Here's how the part is built. I have some questions about the finished solid (model axes, mm). Face numbers are marked on the shaded views. A direction names the side the tool comes from. Give positions to 0.01 mm unless a question says otherwise; leave off trailing zeros. Loops run counter-clockwise (first coordinate to the right, second up) from the corner with the lowest first, then second, coordinate; pieces in that order, holes last. Notation, with made-up numbers: (13, -38) - (51, -38) arc R25 cw to (51, -17) - close; hole circle Ø4 at (62.5, 85). An arc over 180 degrees is marked (long way). Use a Markdown table: item, result.
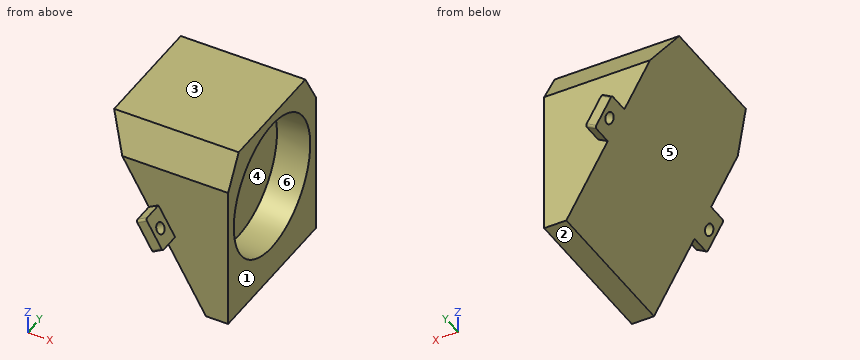
from build123d import *

# Parameters (mm, degrees)
BOSS_EXTRUDE1_DEPTH = 88.9
SKETCH2_R           = 38.735
CUT_EXTRUDE1_DEPTH  = 6.35
SKETCH3_W           = 101.6
SKETCH3_H           = 88.9
SKETCH3_R           = 38.735
BOSS_EXTRUDE2_DEPTH = 12.7
BOSS_EXTRUDE4_DEPTH = 12.7
SKETCH6_R           = 3.175
CUT_EXTRUDE2_DEPTH  = 58.15
BOSS_EXTRUDE5_DEPTH = 12.7
SKETCH8_R           = 3.175
CUT_EXTRUDE3_DEPTH  = 58.15
FILLET1_R           = 1.27
CUT_EXTRUDE4_DEPTH  = 72.35878735


with BuildPart() as part:
    # Sketch1 → Boss-Extrude1 (new body)
    with BuildSketch(Plane(origin=(0, 0, 0), x_dir=(1, 0, 0), z_dir=(0, 1, 0))):
        Polygon((0, 0), (0, 101.6), (-58.65878735, 0), align=None)
    extrude(amount=BOSS_EXTRUDE1_DEPTH)

    # Sketch2 → Cut-Extrude1 (cut)
    with BuildSketch(Plane(origin=(0, 0, 0), x_dir=(0, 0, -1), z_dir=(1, 0, 0))):
        with Locations((44.45, 44.45)):
            Circle(SKETCH2_R)
    extrude(amount=-CUT_EXTRUDE1_DEPTH, mode=Mode.SUBTRACT)

    # Sketch3 → Boss-Extrude2 (add)
    with BuildSketch(Plane(origin=(0, 0, 0), x_dir=(0, 0, -1), z_dir=(1, 0, 0))):
        with Locations((50.8, 44.45)):
            Rectangle(SKETCH3_W, SKETCH3_H)
        with Locations((44.45, 44.45)):
            Circle(SKETCH3_R, mode=Mode.SUBTRACT)
    extrude(amount=BOSS_EXTRUDE2_DEPTH)

    # Sketch5 → Boss-Extrude4 (add)
    with BuildSketch(Plane.XZ):
        Polygon((-23.197585425, -61.42060343), (-32.722585425, -44.922819488), (-27.223324111, -41.747819488), (-17.698324111, -58.24560343), align=None)
    extrude(amount=BOSS_EXTRUDE4_DEPTH)

    # Sketch6 → Cut-Extrude2 (cut, through all)
    with BuildSketch(Plane(origin=(-38.494829198, 0, -22.225), x_dir=(0.5, 0, -0.866025404), z_dir=(0.866025404, 0, 0.5))):
        with Locations((32.068010174, -6.46367916)):
            Circle(SKETCH6_R)
    extrude(amount=-CUT_EXTRUDE2_DEPTH, mode=Mode.SUBTRACT)

    # Sketch7 → Boss-Extrude5 (add)
    with BuildSketch(Plane(origin=(0, 88.9, 0), x_dir=(1, 0, 0), z_dir=(0, 1, 0))):
        Polygon((-23.73378735, 60.491874454), (-18.234526036, 57.316874454), (-27.759526036, 40.819090512), (-33.25878735, 43.994090512), align=None)
    extrude(amount=BOSS_EXTRUDE5_DEPTH)

    # Sketch8 → Cut-Extrude3 (cut, through all)
    with BuildSketch(Plane(origin=(-38.494829198, 0, -22.225), x_dir=(0.5, 0, -0.866025404), z_dir=(0.866025404, 0, 0.5))):
        with Locations((30.995606325, 95.541359592)):
            Circle(SKETCH8_R)
    extrude(amount=-CUT_EXTRUDE3_DEPTH, mode=Mode.SUBTRACT)

    # Fillet1
    fillet1_edges = [part.edges().sort_by_distance(p)[0] for p in [
        (-20.447954768, -12.7, -59.83310343),
        (-29.972954768, -12.7, -43.335319488),
        (-30.509156693, 101.6, -42.406590512),
        (-20.984156693, 101.6, -58.904374454),
    ]]
    fillet(fillet1_edges, radius=FILLET1_R)

    # Sketch9 → Cut-Extrude4 (cut, through all)
    with BuildSketch(Plane(origin=(12.7, 0, 0), x_dir=(0, 0, -1), z_dir=(1, 0, 0))):
        Polygon((18.509160794, 88.9), (0, 78.213731033), (0, 88.9), align=None)
        Polygon((0, 10.686268967), (0, 0), (18.509160794, 0), align=None)
    extrude(amount=-CUT_EXTRUDE4_DEPTH, mode=Mode.SUBTRACT)


solid = part.part
(1) Suppose I cut it at A-A on y = 50.5. Write out the boundary of the cut face in (x, z), plus the area to 3 significant figures.
A:
| item | result |
|---|---|
| outline | (-58.66, 0) - (0, -101.6) - (12.7, -101.6) - (12.7, -82.71) - (-6.35, -82.71) - (-6.35, -6.19) - (12.7, -6.19) - (12.7, 0) - close |
| area | 2,810 mm2 |
(2) Suppose I cut it at B-B on z = -80.5. Write out the boundary of the cut face in (x, y).
A:
| item | result |
|---|---|
| outline | (-12.18, 0) - (12.7, 0) - (12.7, 30.28) - (-6.35, 30.28) - (-6.35, 58.62) - (12.7, 58.62) - (12.7, 88.9) - (-12.18, 88.9) - close |
(3) Will these pins go through, and if not, where does the flat tip stop? pin 1 (18 mm diameter, centred on x = -6, z = -44, fed in from +Y); pin 2 (8 mm diameter, centred on y = 63, z = -69.5, fed in from +X); pin 3 (4 mm diameter, centred on y = 20, z = -62.5, fed in from -X).
A:
| item | result |
|---|---|
| pin 1 | y = 88.9 |
| pin 2 | x = -6.35 |
| pin 3 | x = -23.73 |
(4) We'd pull the mould along Z, two halves only. Please class the marked faces 1, 2, 3 and 4: pulls with the +Z half, pulls with the -Z half, needs draft (parallel to the pull), parting line crosses it, or undercut.
A:
| item | result |
|---|---|
| face 1 | needs draft |
| face 2 | pulls with the -Z half |
| face 3 | pulls with the +Z half |
| face 4 | undercut |
(5) On a 3-axis mill with a long thin cutter (end or side, diameter ignored), from which of +Z, -Z, +X, -X, +Y, -Y can I reach the whole of each face in a straight line? I mean the marked faces 5 and 6. Say none if no direction works.
A:
| item | result |
|---|---|
| face 5 | -Z, -X, +Y, -Y |
| face 6 | +X |
(6) Suppose I cut it at C-C on x = -11. Write out the boundary of the cut face in (y, z).
A:
| item | result |
|---|---|
| outline | (0, -82.55) - (88.9, -82.55) - (88.9, -18.51) - (78.21, 0) - (10.69, 0) - (0, -18.51) - close |
(7) If I drill on line 1 (Y direction, x = 7.75, z = -44.45) (3 decimals); line 2 (Z direction, x = 5, y = 44); line 3 (Y direction, x = 2, z = -65), over which ranges is the centre line in solid material (lowest first)?
A:
| item | result |
|---|---|
| line 1 | 0 to 5.715, 83.185 to 88.9 |
| line 2 | -101.6 to -83.18, -5.72 to 0 |
| line 3 | 0 to 11.62, 77.28 to 88.9 |
